```python
from build123d import *

# Parameters (mm, degrees)
F0_W         = 55
F0_H         = 23
F1_DEPTH     = 60
F2_T         = 2
F3_T1_DEPTH  = 63.5
F3_T3_DEPTH  = 25
F3_T5_DEPTH  = 57
F3_S9_W      = 1
F3_S9_H      = 1
F3_T10_DEPTH = 1
F3_S15_W     = 1
F3_S15_H     = 1
F3_T16_DEPTH = 1
F3_S21_W     = 1
F3_S21_H     = 1
F3_T22_DEPTH = 1
F3_S27_W     = 1
F3_S27_H     = 1
F3_T28_DEPTH = 1
F4_R         = 0.7


# Not quite as in the source:
# - a fillet or chamfer that OpenCascade refuses, or shapes differently, is made with other operations: its cross-section is extruded or revolved along the edge and cut away or added


with BuildPart() as f1:
    # F0 (on Top) → F1 (new body)
    with BuildSketch(Plane.XY):
        Rectangle(F0_W, F0_H)
    extrude(amount=F1_DEPTH)

    # F2
    f2_openings = [f1.faces().sort_by_distance(p)[0] for p in [
        (0, 0, 60),
    ]]
    offset(amount=F2_T, openings=f2_openings, kind=Kind.INTERSECTION)

    # F3: fillet of radius 1 on 8 edges, made by hand

    # F3_s2 → F3_t1 (cut)
    with BuildSketch(Plane.XY.offset(-1)):
        with BuildLine():
            ThreePointArc((29.5, -12.5), (29.2071067812, -13.2071067812), (28.5, -13.5))
            Line((28.5, -13.5), (29.5, -13.5))
            Line((29.5, -13.5), (29.5, -12.5))
        make_face()
        with BuildLine():
            ThreePointArc((29.5, 12.5), (29.2071067812, 13.2071067812), (28.5, 13.5))
            Line((28.5, 13.5), (29.5, 13.5))
            Line((29.5, 13.5), (29.5, 12.5))
        make_face()
        with BuildLine():
            ThreePointArc((-28.5, 13.5), (-29.2071067812, 13.2071067812), (-29.5, 12.5))
            Line((-29.5, 12.5), (-29.5, 13.5))
            Line((-29.5, 13.5), (-28.5, 13.5))
        make_face()
        with BuildLine():
            ThreePointArc((-29.5, -12.5), (-29.2071067812, -13.2071067812), (-28.5, -13.5))
            Line((-28.5, -13.5), (-29.5, -13.5))
            Line((-29.5, -13.5), (-29.5, -12.5))
        make_face()
    extrude(amount=F3_T1_DEPTH, mode=Mode.SUBTRACT)

    # F3_s4 → F3_t3 (cut)
    with BuildSketch(Plane.XZ.offset(-12.5)):
        with BuildLine():
            ThreePointArc((29.5, -1), (29.2071067812, -1.7071067812), (28.5, -2))
            Line((28.5, -2), (29.5, -2))
            Line((29.5, -2), (29.5, -1))
        make_face()
        with BuildLine():
            ThreePointArc((-29.5, -1), (-29.2071067812, -1.7071067812), (-28.5, -2))
            Line((-28.5, -2), (-29.5, -2))
            Line((-29.5, -2), (-29.5, -1))
        make_face()
    extrude(amount=F3_T3_DEPTH, mode=Mode.SUBTRACT)

    # F3_s6 → F3_t5 (cut)
    with BuildSketch(Plane.YZ.offset(-28.5)):
        with BuildLine():
            ThreePointArc((13.5, -1), (13.2071067812, -1.7071067812), (12.5, -2))
            Line((12.5, -2), (13.5, -2))
            Line((13.5, -2), (13.5, -1))
        make_face()
        with BuildLine():
            ThreePointArc((-13.5, -1), (-13.2071067812, -1.7071067812), (-12.5, -2))
            Line((-12.5, -2), (-13.5, -2))
            Line((-13.5, -2), (-13.5, -1))
        make_face()
    extrude(amount=F3_T5_DEPTH, mode=Mode.SUBTRACT)


with BuildPart() as f3_tool8:
    # F3_s9 → F3_t10 (new body)
    with BuildSketch(Plane.XZ.offset(12.5)):
        with Locations((29, -1.5)):
            Rectangle(F3_S9_W, F3_S9_H)
    extrude(amount=F3_T10_DEPTH)

    # F3_s11 → F3_t12 (revolve, cut)
    with BuildSketch(Plane(origin=(28.5, -12.5, -1), x_dir=(-0.7071067812, 0, 0.7071067812), z_dir=(0.7071067812, 0, 0.7071067812))):
        with BuildLine():
            ThreePointArc((0, -1), (1, 0), (0, 1))
            Line((0, 1), (0, -1))
        make_face()
    revolve(axis=Axis((28.5, -12.5, -1), (0, -1, 0)), mode=Mode.SUBTRACT)


with BuildPart() as f1_1:
    add(f1.part)

    # F3_t7: cut F3_tool8
    add(f3_tool8.part, mode=Mode.SUBTRACT)


with BuildPart() as f3_tool14:
    # F3_s15 → F3_t16 (new body)
    with BuildSketch(Plane.XY.offset(-1)):
        with Locations((29, 13)):
            Rectangle(F3_S15_W, F3_S15_H)
    extrude(amount=-F3_T16_DEPTH)

    # F3_s17 → F3_t18 (revolve, cut)
    with BuildSketch(Plane(origin=(28.5, 12.5, -1), x_dir=(-0.7071067812, -0.7071067812, 0), z_dir=(0.7071067812, -0.7071067812, 0))):
        with BuildLine():
            ThreePointArc((0, -1), (1, 0), (0, 1))
            Line((0, 1), (0, -1))
        make_face()
    revolve(axis=Axis((28.5, 12.5, -1), (0, 0, -1)), mode=Mode.SUBTRACT)


with BuildPart() as f1_2:
    add(f1_1.part)

    # F3_t13: cut F3_tool14
    add(f3_tool14.part, mode=Mode.SUBTRACT)


with BuildPart() as f3_tool20:
    # F3_s21 → F3_t22 (new body)
    with BuildSketch(Plane.YZ.offset(-28.5)):
        with Locations((13, -1.5)):
            Rectangle(F3_S21_W, F3_S21_H)
    extrude(amount=-F3_T22_DEPTH)

    # F3_s23 → F3_t24 (revolve, cut)
    with BuildSketch(Plane(origin=(-28.5, 12.5, -1), x_dir=(0, -0.7071067812, 0.7071067812), z_dir=(0, -0.7071067812, -0.7071067812))):
        with BuildLine():
            ThreePointArc((0, -1), (1, 0), (0, 1))
            Line((0, 1), (0, -1))
        make_face()
    revolve(axis=Axis((-28.5, 12.5, -1), (-1, 0, 0)), mode=Mode.SUBTRACT)


with BuildPart() as f1_3:
    add(f1_2.part)

    # F3_t19: cut F3_tool20
    add(f3_tool20.part, mode=Mode.SUBTRACT)


with BuildPart() as f3_tool26:
    # F3_s27 → F3_t28 (new body)
    with BuildSketch(Plane.YZ.offset(-28.5)):
        with Locations((-13, -1.5)):
            Rectangle(F3_S27_W, F3_S27_H)
    extrude(amount=-F3_T28_DEPTH)

    # F3_s29 → F3_t30 (revolve, cut)
    with BuildSketch(Plane(origin=(-28.5, -12.5, -1), x_dir=(0, 0.7071067812, 0.7071067812), z_dir=(0, -0.7071067812, 0.7071067812))):
        with BuildLine():
            ThreePointArc((0, -1), (1, 0), (0, 1))
            Line((0, 1), (0, -1))
        make_face()
    revolve(axis=Axis((-28.5, -12.5, -1), (-1, 0, 0)), mode=Mode.SUBTRACT)


with BuildPart() as f1_4:
    add(f1_3.part)

    # F3_t25: cut F3_tool26
    add(f3_tool26.part, mode=Mode.SUBTRACT)

    # F4
    f4_edges = [f1_4.edges().sort_by_distance(p)[0] for p in [
        (0, -11.5, 60),
        (27.5, 0, 60),
        (0, 11.5, 60),
        (-27.5, 0, 60),
        (0, 13.5, 60),
        (0, -13.5, 60),
        (-29.5, 0, 60),
        (29.5, 0, 60),
        (-29.207107, 13.207107, 60),
        (29.207107, 13.207107, 60),
        (29.207107, -13.207107, 60),
        (-29.207107, -13.207107, 60),
    ]]
    fillet(f4_edges, radius=F4_R)


solid = f1_4.part
```
Here's how the part is built. I have some questions about the finished solid (model axes, mm). A direction names the side the tool comes from. Coordinates: 2 decimals unless noted, no trailing zeros. Write each loop counter-clockwise with the first axis right and the second up, starting at its lowest first coordinate (ties: lowest second). Pieces come first, ordered by that corner, then holes. Notation, with made-up numbers: (47.25, 41) -> (80.25, 41) arc R26 cw to (80.25, 74) -> close; hole circle Ø10 at (14.25, 62.5). An arc over 180 degrees is marked (long way). Use a Markdown table: item, result. Add a question column.
(1) Please list where these lines run through material, in increasing order: line 1 (Y direction, x = -10, z = 56); line 2 (X direction, y = -2.25, z = 23.5); line 3 (Z direction, x = -23, y = -8.75).
(2) If we section it at B-B, the plane y = -8.75: Write out the boundary of the cut face in (x, z).
(3) We'd pull the mould along Y, two halves only. Please class faces 3 (the flat face through (0, -13.5, 29)), 4 (the flat face through (-29.5, 0, 29)), 5 (the flat face through (27.5, 0, 29)), 6 (the flat face through (0, -11.5, 29)): +Y half, -Y half, draft (parallel to the pull), parting line (faces both ways), or undercut.
(4) If we section it at A-A, the plane z = 3: Write out the boundary of the cut face in (x, y).
(5) If we section it at C-C, the plane x = 1: Write out the boundary of the cut face in (y, z).
(6) For faces 1 (the flat face through (0, 0, -2)), 2 (the flat face through (0, 0, 0)), which set-ups out of +Z, -Z, +X, -X, +Y, -Y let a thin tool reach every point of the face, with its end or its side?
Outcome:
| question | item | result |
|---|---|---|
| 1 | line 1 | y = -13.5 to -11.5, 11.5 to 13.5 |
| 1 | line 2 | x = -29.5 to -27.5, 27.5 to 29.5 |
| 1 | line 3 | z = -2 to 0 |
| 2 | outline | (-29.5, -1) arc R1 ccw to (-28.5, -2) -> (28.5, -2) arc R1 ccw to (29.5, -1) -> (29.5, 59.3) arc R0.7 ccw to (28.8, 60) -> (28.2, 60) arc R0.7 ccw to (27.5, 59.3) -> (27.5, 0) -> (-27.5, 0) -> (-27.5, 59.3) arc R0.7 ccw to (-28.2, 60) -> (-28.8, 60) arc R0.7 ccw to (-29.5, 59.3) -> close |
| 3 | face 3 | -Y half |
| 3 | face 4 | draft |
| 3 | face 5 | undercut |
| 3 | face 6 | undercut |
| 4 | outline | (-29.5, -12.5) arc R1 ccw to (-28.5, -13.5) -> (28.5, -13.5) arc R1 ccw to (29.5, -12.5) -> (29.5, 12.5) arc R1 ccw to (28.5, 13.5) -> (-28.5, 13.5) arc R1 ccw to (-29.5, 12.5) -> close; hole (-27.5, -11.5) -> (27.5, -11.5) -> (27.5, 11.5) -> (-27.5, 11.5) -> close |
| 5 | outline | (-13.5, -1) arc R1 ccw to (-12.5, -2) -> (12.5, -2) arc R1 ccw to (13.5, -1) -> (13.5, 59.3) arc R0.7 ccw to (12.8, 60) -> (12.2, 60) arc R0.7 ccw to (11.5, 59.3) -> (11.5, 0) -> (-11.5, 0) -> (-11.5, 59.3) arc R0.7 ccw to (-12.2, 60) -> (-12.8, 60) arc R0.7 ccw to (-13.5, 59.3) -> close |
| 6 | face 1 | -Z, +X, -X, +Y, -Y |
| 6 | face 2 | +Z |
